Input: part model. Units: mm. Frame: model coordinates. A direction names the side the tool comes from. Give positions to 0.01 mm unless a question says otherwise; leave off trailing zeros. Order: outer loops, then holes, each group sorted by start corner. A loop starts at its lowest first (then second) coordinate and runs counter-clockwise, first axis right, second up. Notation, with made-up numbers: M 47.5,-8.75 L 66.5,-8.75 A24 ccw 66.5,27.25 Z; hole C 89,42 d4. An arc over 180 degrees is marked long. Use a Markdown table: item, result.
from build123d import *

# Parameters (mm, degrees)
F1_DEPTH = 63.5
F0_W     = 20.7627861344
F0_H     = 19.05
F2_DEPTH = 25.4
F3_DEPTH = 6.35
F5_R     = 12.7


with BuildPart() as f1:
    # F0 (on Front) → F1 (new body, symmetric)
    with BuildSketch(Plane.XZ):
        Polygon((-41.275, -9.525), (41.275, -9.525), (41.275, 9.525), (22.225, 9.525), (-41.275, 9.525), align=None)
    extrude(amount=F1_DEPTH, both=True)

    # F0 (on Front) → F2 (join, symmetric)
    with BuildSketch(Plane.XZ):
        with BuildLine():
            Line((22.225, 9.525), (41.275, 9.525))
            Line((41.275, 9.525), (41.275, 27.0002))
            ThreePointArc((41.275, 27.0002), (45.9246798487, 38.2255201513), (57.15, 42.8752))
            Line((57.15, 42.8752), (60.325, 42.8752))
            Line((60.325, 42.8752), (60.325, 61.9252))
            Line((60.325, 61.9252), (57.15, 61.9252))
            ThreePointArc((57.15, 61.9252), (32.4542956671, 51.6959043329), (22.225, 27.0002))
            Line((22.225, 27.0002), (22.225, 9.525))
        make_face()
        with Locations((70.7063930672, 52.4002)):
            Rectangle(F0_W, F0_H)
    extrude(amount=F2_DEPTH, both=True)

    # F0 (on Front) → F3 (join, symmetric)
    with BuildSketch(Plane.XZ):
        with BuildLine():
            add(Edge.make_bspline(
                [(-41.275, 9.525), (-4.0282602422, 16.1482468247), (17.7380666137, 62.469098717), (57.15, 61.9252)],
                knots=[0, 0, 0, 0, 111.5045361635, 111.5045361635, 111.5045361635, 111.5045361635], degree=3))
            Line((-41.275, 9.525), (22.225, 9.525))
            Line((22.225, 9.525), (22.225, 27.0002))
            ThreePointArc((22.225, 27.0002), (32.4542956671, 51.6959043329), (57.15, 61.9252))
        make_face()
    extrude(amount=F3_DEPTH, both=True)

    # F0 (on Front) → F4 (revolve)
    with BuildSketch(Plane.XZ):
        Polygon((81.0877861344, 66.675), (81.0877861344, 61.9252), (81.0877861344, 42.8752), (81.0877861344, 38.1), (111.125, 38.1), (111.125, 66.675), align=None)
    revolve(axis=Axis((81.0877861344, 0, 52.4002), (0, 0, 1)))

    # F5
    f5_edges = [f1.edges().sort_by_distance(p)[0] for p in [
        (-41.275, 63.5, 0),
        (-41.275, -63.5, 0),
        (41.275, -63.5, 0),
        (41.275, 63.5, 0),
    ]]
    fillet(f5_edges, radius=F5_R)


solid = f1.part
1) First-contact query: pin 1 Ø12 at (y, z) = (8, 43.5) entering from +X; pin 2 Ø2 at (x, y) = (60, 23) entering from -Z; pin 3 Ø8 at (x, y) = (62.5, -20.5) entering from -Z; pin 4 Ø15.5 at (x, z) = (-15, 37) entering from -Y. Flat tips, straight axial feed; report the tip coordinate or a pass-through.
Response values:
| item | result |
|---|---|
| pin 1 | stops at x = 111.06 |
| pin 2 | stops at z = 42.88 |
| pin 3 | stops at z = 38.1 |
| pin 4 | passes through |
2) Mould query, pull axis X, two halves, no side actions, for faces 6 (the face through (22.225, -16, 18)), 7 (the face through (59, 23, 42.875)), 8 (the face through (1, -35, 9.525)). Classes: released by +X, released by -X, zero draft, split by the parting line, or undercut.
Response values:
| item | result |
|---|---|
| face 6 | released by -X |
| face 7 | undercut |
| face 8 | zero draft |
3) Cut plane B-B on y = -14. Return loops of the section in (x, z) (3 decimals).
Response values:
| item | result |
|---|---|
| outline | M -41.275,-9.525 L 41.275,-9.525 L 41.275,27 A15.875 cw 54.513,42.655 L 54.513,38.1 L 107.663,38.1 L 107.663,66.675 L 54.513,66.675 L 54.513,61.825 A34.925 ccw 22.225,27 L 22.225,9.525 L -41.275,9.525 Z |
4) Cut plane A-A on z = 6.5. Return loops of the section in (x, y) (3 decimals), and give its area (3 significant figures).
Response values:
| item | result |
|---|---|
| outline | M -41.275,-50.8 A12.7 ccw -28.575,-63.5 L 28.575,-63.5 A12.7 ccw 41.275,-50.8 L 41.275,50.8 A12.7 ccw 28.575,63.5 L -28.575,63.5 A12.7 ccw -41.275,50.8 Z |
| area | 10,300 mm² |
5) Material intervals for line 1 (X direction, y = -9, z = 5) (3 decimals); line 2 (Z direction, x = 6.5, y = -38) (3 decimals); line 3 (Y direction, x = -3, z = 18), sorted ascending. Write a range as from..to.
Response values:
| item | result |
|---|---|
| line 1 | x = -41.275..41.275 |
| line 2 | z = -9.525..9.525 |
| line 3 | y = -6.35..6.35 |
6) Cut plane C-C on y = -48. Return loops of the section in (x, z) (3 decimals), and give its area (3 significant figures).
Response values:
| item | result |
|---|---|
| outline | M -41.275,-9.525 L 41.275,-9.525 L 41.275,9.525 L -41.275,9.525 Z |
| area | 1,570 mm² |
7) Reachability of faces 1 (the face through (82, 0, 38.1)), 2 (the face through (59, -23, 61.925)), 3 (the face through (81, 0, 66.675)), 4 (the face through (59, -23, 42.875)), 5 (the face through (59, 23, 61.925)) from +Z, -Z, +X, -X, +Y, -Y: full face, straight path, thin tool, end or side. Return the list, or none.
Response values:
| item | result |
|---|---|
| face 1 | -Z, +X, +Y, -Y |
| face 2 | +Z, -X, -Y |
| face 3 | +Z, +X, -X, +Y, -Y |
| face 4 | -Z, -Y |
| face 5 | +Z, -X, +Y |
